Here's the drawing with two shaded views (mm, measured from the low corner). I have some questions. Give positions to 0.01 mm unless a question says otherwise; leave off trailing zeros. Loops run counter-clockwise (first coordinate to the right, second up) from the corner with the lowest first, then second, coordinate; pieces in that order, holes last.
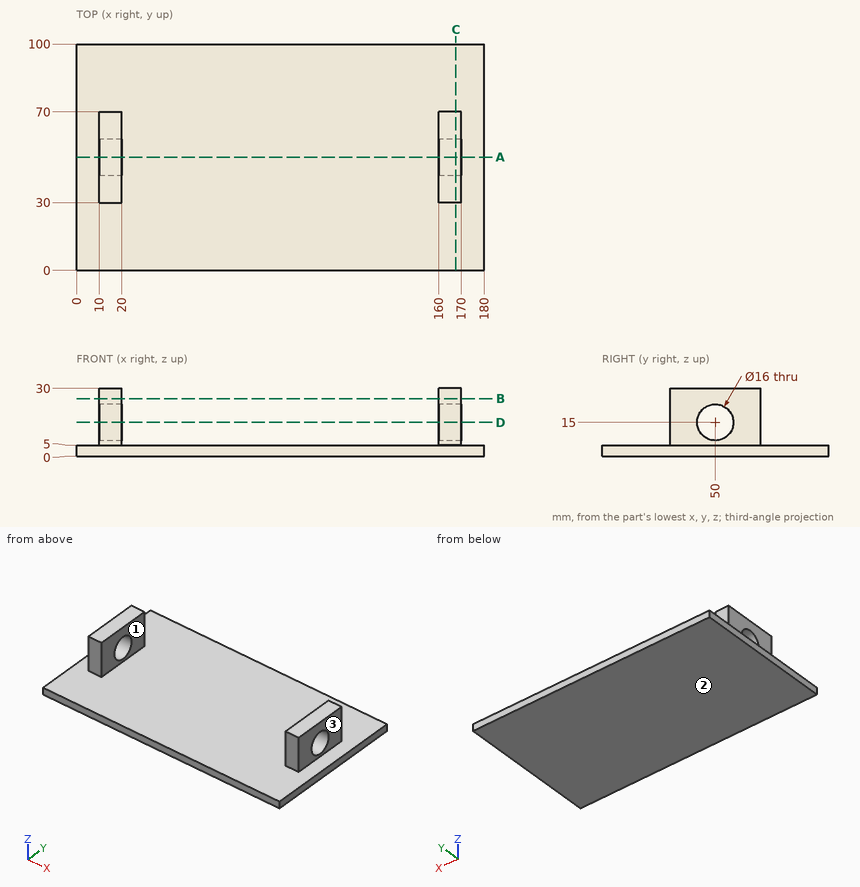
(1) Suppose I cut it at B-B on z = 25.5. List the corners of the cut face in (x, y) for me, plus the area to 3 significant figures.
Returned:
outline: (10, 30) - (20, 30) - (20, 70) - (10, 70) - close; (160, 30) - (170, 30) - (170, 70) - (160, 70) - close
area: 800 mm2
(2) Suppose I cut it at C-C on x = 167.5. List the corners of the cut face in (y, z) for me.
Returned:
outline: (0, 0) - (100, 0) - (100, 5) - (70, 5) - (70, 30) - (30, 30) - (30, 5) - (0, 5) - close; hole circle Ø16 at (50, 15)
(3) Suppose I cut it at A-A on y = 50. List the corners of the cut face in (x, z) for me, plus the area to 3 significant figures.
Returned:
outline: (0, 0) - (180, 0) - (180, 5) - (170, 5) - (170, 7) - (160, 7) - (160, 5) - (20, 5) - (20, 7) - (10, 7) - (10, 5) - (0, 5) - close; (10, 23) - (20, 23) - (20, 30) - (10, 30) - close; (160, 23) - (170, 23) - (170, 30) - (160, 30) - close
area: 1,080 mm2
(4) Suppose I cut it at D-D on z = 15. List the corners of the cut face in (x, y) for me.
Returned:
outline: (10, 30) - (20, 30) - (20, 42) - (10, 42) - close; (10, 58) - (20, 58) - (20, 70) - (10, 70) - close; (160, 30) - (170, 30) - (170, 42) - (160, 42) - close; (160, 58) - (170, 58) - (170, 70) - (160, 70) - close
(5) Please list where these lines run through material, in increasing order: probe 1 along X at (y, z) = (51.5, 25.75); probe 2 along Z at (x, y) = (12.75, 50); probe 3 along Y at (x, z) = (11, 14.75).
Returned:
probe 1: x = 10 to 20, 160 to 170
probe 2: z = 0 to 7, 23 to 30
probe 3: y = 30 to 42, 58 to 70
(6) Thinking about a two-plate mould opening in X: for the marked faces 1, 2 and 3, which applies, pulls with the +X half, pulls with the -X half, needs draft (parallel to the pull), parting line crosses it, or undercut?
Returned:
face 1: undercut
face 2: needs draft
face 3: pulls with the +X half
(7) Will these pins go through, and if not, where does the flat tip stop? P1, Ø11, axis at x = 165, z = 15.5, coming from the +Y side; P2, Ø8, axis at x = 114, z = 6, coming from the -Y side; P3, Ø3, axis at x = 13.5, z = 21.5, coming from the -Y side; P4, Ø8, axis at x = 30, y = 60, coming from the +Z side.
Returned:
P1: stops at y = 70
P2: stops at y = 0
P3: stops at y = 30
P4: stops at z = 5
